The figure shows three views and two pictorial views of one solid part (mm, origin at its lowest corner). Answer the questions. Give positions to 0.01 mm unless a question says otherwise; leave off trailing zeros. Loops run counter-clockwise (first coordinate to the right, second up) from the corner with the lowest first, then second, coordinate; pieces in that order, holes last. Notation, with made-up numbers: M 79.25,-0.5 L 135.25,-0.5 A17 cw 135.25,32.5 Z; hole C 51,10.5 d4. An arc over 180 degrees is marked long. Write item = value, one per line. Start each with the question number.
1. Section B-B on x = 1.05 is taken. Determine the outline of the cut face in (y, z).
2. Consider L1, parallel to Y at x = 1.7, z = 22.56; L2, parallel to Y at x = 0.8, z = 40.5; L3, parallel to Z at x = 1, y = 27. Determine where each line is inside the solid, lowest interval first. Write a range as [from, to].
3. Section A-A on y = 7.91 is taken. Determine the outline of the cut face in (x, z), plus the area to 3 significant figures.
4. Flat-ended cylindrical pins translate along their axes: pin 1 Ø2.5 at (y, z) = (7.91, 22.56) entering from +X; pin 2 Ø1.5 at (x, y) = (1.5, 24.5) entering from +Z. Find the tip coordinate at first contact, or state that the pin passes through.
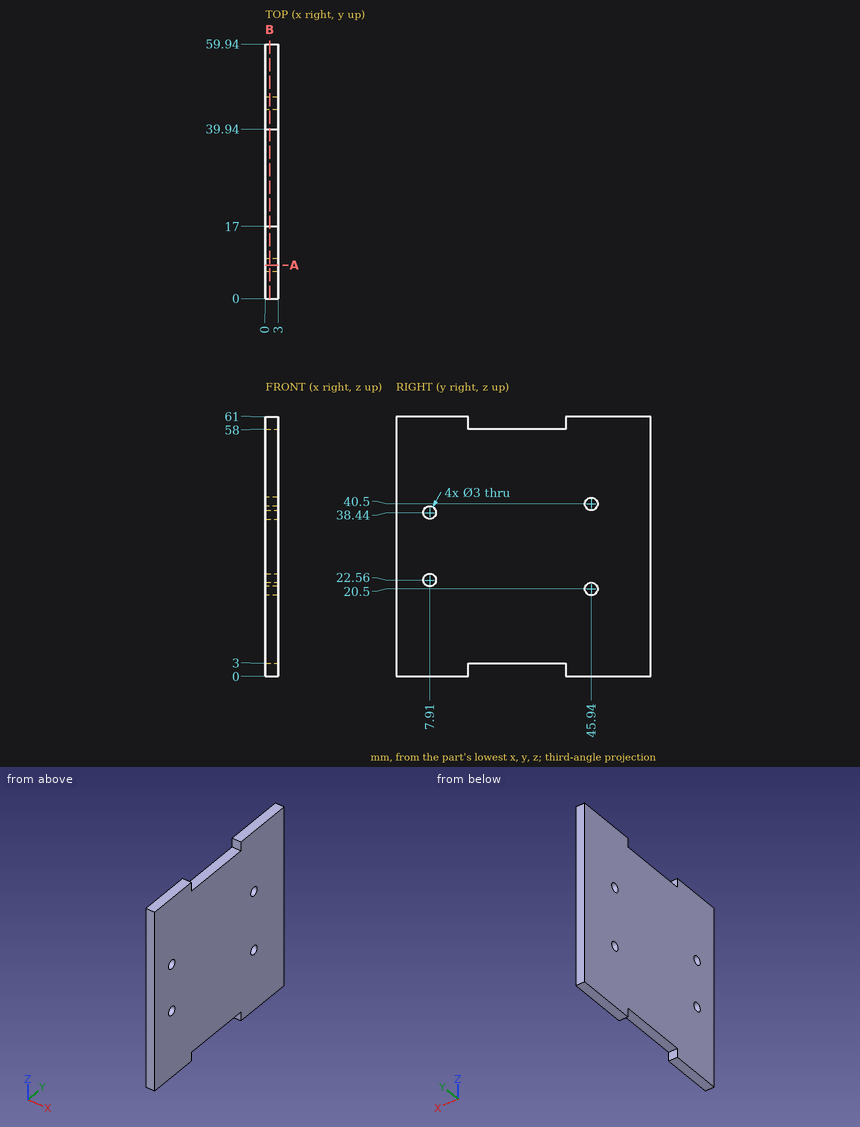
Verdict:
q1.outline = M 0,0 L 17,0 L 17,3 L 39.94,3 L 39.94,0 L 59.94,0 L 59.94,61 L 39.94,61 L 39.94,58 L 17,58 L 17,61 L 0,61 Z; hole C 7.91,22.56 d3; hole C 7.91,38.44 d3; hole C 45.94,20.5 d3; hole C 45.94,40.5 d3
q2.L1 = [0, 6.41], [9.41, 59.94]
q2.L2 = [0, 44.44], [47.44, 59.94]
q2.L3 = [3, 58]
q3.outline = M 0,0 L 3,0 L 3,21.06 L 0,21.06 Z; M 0,24.06 L 3,24.06 L 3,36.94 L 0,36.94 Z; M 0,39.94 L 3,39.94 L 3,61 L 0,61 Z
q3.area = 165 mm2
q4.pin_1 = through
q4.pin_2 = 58
